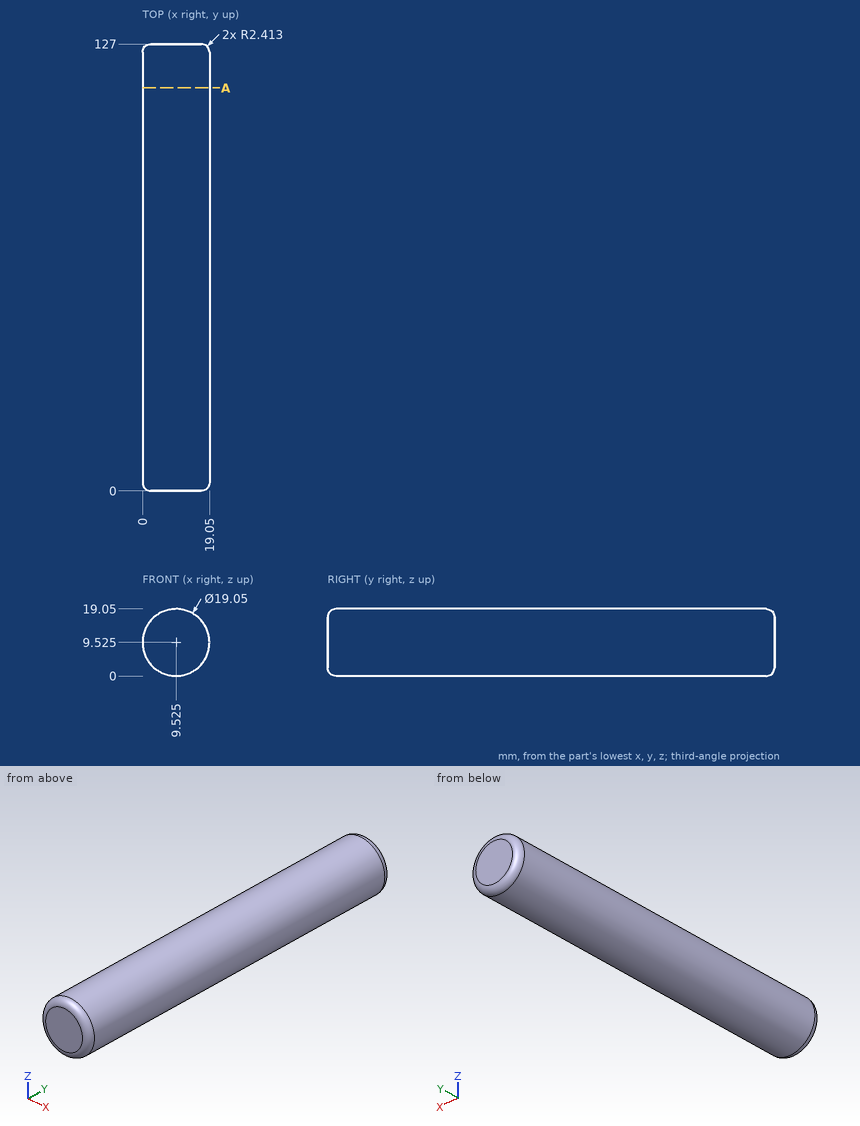
Geometry: see drawing. Coordinates: mm, zero at the bounding-box minimum. Give positions to 0.01 mm unless a question says otherwise; leave off trailing zeros. Order: outer loops, then holes, each group sorted by start corner. A loop starts at its lowest first (then second) coordinate and runs counter-clockwise, first axis right, second up. Notation, with made-up numbers: M 78.5,-13.75 L 136.5,-13.75 A34 cw 136.5,21.25 Z; hole C 56.25,44 d6. An arc over 180 degrees is marked long. Answer as CSV lines item,"result". Start each with the question number.
1) Cut plane A-A (y = 114.5). Output: boundary loops of the cut face in (x, z) (3 decimals).
2) First-contact query: P1, Ø1.5, axis at y = 32.5, z = 13, coming from the +X side; P2, Ø8, axis at x = 3, y = 98.5, coming from the +Z side; P3, Ø2, axis at y = 44, z = 12.5, coming from the -X side. Flat tips, straight axial feed; report the tip coordinate or a pass-through.
3) Line query: line 1 (Z direction, x = 17.5, y = 9); line 2 (Z direction, x = 13, y = 24); line 3 (Y direction, x = 15.75, z = 15.5). Output: solid intervals per line, ascending. Write a range as from..to.
Findings below:
1,outline,"C 9.525,9.525 d19.05"
2,P1,"stops at x = 18.65"
2,P2,"stops at z = 18.71"
2,P3,"stops at x = 0.21"
3,line 1,"z = 4.32..14.73"
3,line 2,"z = 0.66..18.39"
3,line 3,"y = 0.54..126.46"
